Part model, mm, in its own coordinate system. A direction names the side the tool comes from. Round coordinates to 2 decimals unless told otherwise and drop trailing zeros. Order: outer loops, then holes, each group sorted by start corner. A loop starts at its lowest first (then second) coordinate and runs counter-clockwise, first axis right, second up. Notation, with made-up numbers: (38, 20) - (85, 20) arc R24 ccw to (85, 31) - close; hole circle Ø5 at (51, 59.25). An arc over 180 degrees is marked (long way). Return JSON: item names as keys, results as strings. Group by question number.
Item 1: Probe probe 1 along X at (y, z) = (19, -0.5); probe 2 along Y at (x, z) = (39.5, 13.5); probe 3 along Y at (x, z) = (5.5, 7) (3 decimals). List the from-to ranges inside material, lowest first.
Item 2: Saw through at C-C on y = -7.5. List the corners of the cut face in (x, z) (3 decimals), and give its area (3 significant figures).
Item 3: Saw through at B-B on x = 100. List the corners of the cut face in (y, z) (3 decimals).
Item 4: Tool access for faces 1 (the face through (19.05, -10, 11)), 2 (the face through (97, 0, 0)), 3 (the face through (28, 19.05, 27)), 4 (the face through (9, -6, 26.924)): list every direction of +Z, -Z, +X, -X, +Y, -Y with a clear straight run to the whole face (end or side of a thin tool).
Item 5: Saw through at A-A on y = 14.5. List the corners of the cut face in (x, z) (3 decimals).
Item 6: Saw through at D-D on x = 17. List the corners of the cut face in (y, z) (3 decimals).
Item 7: Two-plate mould, pull along Z, no slides. Class faces 5 (the face through (80.722, 10.153, 11.889)), 6 (the face through (7.411, 9.392, 41.524)), 7 (the face through (9.658, -17.239, 25.014)): released by +Z, released by -Z, zero draft, split by the parting line, or undercut.
Item 8: Drop flat-ended pins along their axis: pin 1 (10 mm diameter, centred on y = 18.5, z = 21.5, fed in from -X); pin 2 (6.5 mm diameter, centred on x = 7.5, y = -8, fed in from +Z); pin 3 (2 mm diameter, centred on y = 15.5, z = 36, fed in from +X); pin 4 (6 mm diameter, centred on x = 56, y = 22.5, fed in from -Z). Give the stop position or say it passes through.
```python
from build123d import *

# Parameters (mm, degrees)
F0_R       = 3.556
F1_DEPTH   = 19.05
F2_W       = 19.05
F2_H       = 26.924
F2_R       = 3.175
F3_DEPTH   = 19.05
F4_R       = 6.35
F6_W       = 73.152
F6_H       = 12.7
F7_DEPTH   = 15.875
F8_R       = 14.2875
F9_DEPTH   = 12.7
F8_R_2     = 6.6675
F10_DEPTH  = 11.0998
F12_DEPTH  = 3.175
F12_FACE_W = 12.7
F12_FACE_H = 57.15
F13_DEPTH  = 15.875


with BuildPart() as f1:
    # F0 (on Front) → F1 (new body)
    with BuildSketch(Plane.XZ):
        Polygon((0, 47.6504), (0, 0), (73.152, 0), (73.152, 12.7), (28.702, 47.6504), align=None)
        with Locations((7.874, 37.9984)):
            Circle(F0_R, mode=Mode.SUBTRACT)
    extrude(amount=-F1_DEPTH)

    # F2 (on Right) → F3 (join)
    with BuildSketch(Plane.YZ):
        with Locations((-9.525, 13.462)):
            Rectangle(F2_W, F2_H)
        with Locations((-9.525, 16.002)):
            Circle(F2_R, mode=Mode.SUBTRACT)
    extrude(amount=F3_DEPTH)

    # F4
    f4_edges = [f1.edges().sort_by_distance(p)[0] for p in [
        (9.525, -19.05, 26.924),
    ]]
    fillet(f4_edges, radius=F4_R)

    # F6 (on offset) → F7 (join)
    with BuildSketch(Plane.XZ.offset(-19.05)):
        with Locations((36.576, 6.35)):
            Rectangle(F6_W, F6_H)
    extrude(amount=-F7_DEPTH)

    # F8 (on Top) → F9 (join)
    with BuildSketch(Plane.XY):
        Polygon((73.152, 34.925), (73.152, 0), (73.152, -22.225), (117.602, -22.225), (117.602, 9.525), (117.602, 34.925), align=None)
        with Locations((94.996, 9.525)):
            Circle(F8_R, mode=Mode.SUBTRACT)
    extrude(amount=F9_DEPTH)

    # F8 (on Top) → F10 (join)
    with BuildSketch(Plane.XY):
        with Locations((94.996, 9.525)):
            Circle(F8_R)
        with Locations((94.996, 9.525)):
            Circle(F8_R_2, mode=Mode.SUBTRACT)
    extrude(amount=F10_DEPTH)

    # F11 (on Top) → F12 (join)
    with BuildSketch(Plane.XY):
        Polygon((76.2, 34.925), (63.5, 34.925), (63.5, 0), (63.5, -22.225), (76.2, -22.225), align=None)
    extrude(amount=-F12_DEPTH)

    # F12_face (on face) → F13 (join)
    with BuildSketch(Plane(origin=(69.85, 6.35, -3.175), x_dir=(1, 0, 0), z_dir=(0, 0, -1))):
        Rectangle(F12_FACE_W, F12_FACE_H)
    extrude(amount=-F13_DEPTH)


solid = f1.part
```
Filled in:
{
 "1": {"probe 1": "x = 63.5 to 76.2", "probe 2": "y = 0 to 19.05", "probe 3": "y = -19.05 to 34.925"},
 "2": {"outline": "(0, 0) - (19.05, 0) - (19.05, 13.557) - (0, 13.557) - close; (0, 18.447) - (19.05, 18.447) - (19.05, 26.924) - (0, 26.924) - close; (63.5, -3.175) - (76.2, -3.175) - (76.2, 0) - (117.602, 0) - (117.602, 12.7) - (63.5, 12.7) - close", "area": "1,150 mm^2"},
 "3": {"outline": "(-22.225, 0) - (5.119, 0) - (5.119, 11.1) - (-3.858, 11.1) - (-3.858, 12.7) - (-22.225, 12.7) - close; (13.931, 0) - (34.925, 0) - (34.925, 12.7) - (22.908, 12.7) - (22.908, 11.1) - (13.931, 11.1) - close"},
 "4": {"face 1": "+Z, -Z, -Y", "face 2": "-Z, +X, +Y, -Y", "face 3": "+Z, +X, -X, +Y", "face 4": "+Z, +X, -X, -Y"},
 "5": {"outline": "(0, 0) - (63.5, 0) - (63.5, -3.175) - (76.2, -3.175) - (76.2, 0) - (90.557, 0) - (90.557, 11.1) - (81.603, 11.1) - (81.603, 12.7) - (73.152, 12.7) - (28.702, 47.65) - (0, 47.65) - close; (99.435, 0) - (117.602, 0) - (117.602, 12.7) - (108.389, 12.7) - (108.389, 11.1) - (99.435, 11.1) - close; hole circle Ø7.112 at (7.874, 37.998)"},
 "6": {"outline": "(-19.05, 0) - (34.925, 0) - (34.925, 12.7) - (19.05, 12.7) - (19.05, 47.65) - (0, 47.65) - (0, 26.924) - (-12.7, 26.924) arc R6.35 ccw to (-19.05, 20.574) - close; hole circle Ø6.35 at (-9.525, 16.002)"},
 "7": {"face 5": "zero draft", "face 6": "undercut", "face 7": "released by +Z"},
 "8": {"pin 1": "stops at x = 0", "pin 2": "stops at z = 26.92", "pin 3": "stops at x = 44.79", "pin 4": "stops at z = 0"}
}
